The listing builds one solid part. Answer for the finished solid, in the listing's coordinates (mm). Coordinates: 2 decimals unless noted, no trailing zeros. Write each loop counter-clockwise with the first axis right and the second up, starting at its lowest first coordinate (ties: lowest second). Pieces come first, ordered by that corner, then holes. Notation, with made-up numbers: M 23.25,14.25 L 40.25,14.25 A36 cw 40.25,48.25 Z; hole C -40,77.5 d9. An arc over 180 degrees is marked long. Answer as CSV lines item,"result". Start each with the question number.
```python
from build123d import *

# Parameters (mm, degrees)
SKETCH_1_W             = 32.7
SKETCH_1_H             = 29
SKETCH_1_R             = 1.5
EXTRUDE_1_DEPTH        = 3
CHAMFER_1_SIZE         = 3
EXTRUDE_2_DEPTH        = 3
CHAMFER_2_SIZE         = 9.5
EXTRUDE_3_DEPTH        = 3
SKETCH_6_R             = 1.6
CUT_EXTRUDE_2_DEPTH    = 4
CUT_EXTRUDE_4_DEPTH    = 10
FILLET_2_R             = 1
FILLET_2_OF_MIRROR_1_R = 1


with BuildPart() as part:
    # 草图1 → 凸台-拉伸1 (new body)
    with BuildSketch(Plane.XY):
        Rectangle(SKETCH_1_W, SKETCH_1_H)
        with Locations((-14.35, -10)):
            Circle(SKETCH_1_R, mode=Mode.SUBTRACT)
        with Locations((-14.35, 10)):
            Circle(SKETCH_1_R, mode=Mode.SUBTRACT)
        with Locations((14.35, 10)):
            Circle(SKETCH_1_R, mode=Mode.SUBTRACT)
        with Locations((14.35, -10)):
            Circle(SKETCH_1_R, mode=Mode.SUBTRACT)
        with Locations((-14.35, 0)):
            Circle(SKETCH_1_R, mode=Mode.SUBTRACT)
        with Locations((14.35, 0)):
            Circle(SKETCH_1_R, mode=Mode.SUBTRACT)
    extrude(amount=EXTRUDE_1_DEPTH)

    # 倒角1
    chamfer_1_edges = [part.edges().sort_by_distance(p)[0] for p in [
        (16.35, -14.5, 1.5),
        (-16.35, -14.5, 1.5),
        (-16.35, 14.5, 1.5),
        (16.35, 14.5, 1.5),
    ]]
    chamfer(chamfer_1_edges, length=CHAMFER_1_SIZE)

    # 草图3 → 凸台-拉伸2 (add)
    with BuildSketch(Plane.XY.offset(3)):
        Polygon((-13.35, 14.5), (-68.5, 14.5), (-68.5, -14.5), (-13.35, -14.5), (-16.35, -11.5), (-16.35, 11.5), align=None)
        Polygon((68.5, 14.5), (13.35, 14.5), (16.35, 11.5), (16.35, -11.5), (13.35, -14.5), (68.5, -14.5), align=None)
    extrude(amount=-EXTRUDE_2_DEPTH)

    # 倒角2
    chamfer_2_edges = [part.edges().sort_by_distance(p)[0] for p in [
        (-68.5, -14.5, 1.5),
        (-68.5, 14.5, 1.5),
        (68.5, -14.5, 1.5),
        (68.5, 14.5, 1.5),
    ]]
    chamfer(chamfer_2_edges, length=CHAMFER_2_SIZE)

    # 草图4 → 凸台-拉伸3 (add)
    with BuildSketch(Plane(origin=(0, 0, 0), x_dir=(-1, 0, 0), z_dir=(0, 0, -1))):
        Polygon((-59, -14.5), (-53, -20.5), (53, -20.5), (59, -14.5), align=None)
    extrude(amount=-EXTRUDE_3_DEPTH)

    # 草图6 → 切除-拉伸2 (cut, through all)
    with BuildSketch(Plane(origin=(0, 0, 0), x_dir=(-1, 0, 0), z_dir=(0, 0, -1))):
        with Locations((-63.5, 0)):
            Circle(SKETCH_6_R)
    cut_extrude_2 = extrude(amount=-CUT_EXTRUDE_2_DEPTH, mode=Mode.SUBTRACT)

    # 草图7 → 切除-拉伸4 (cut)
    with BuildSketch(Plane(origin=(0, 0, 0), x_dir=(-1, 0, 0), z_dir=(0, 0, -1))):
        Polygon((-57, 11.5), (-65.5, 3), (-57.621320344, 3), (-49.121320344, 11.5), align=None)
        Polygon((-57.621320344, -3), (-65.5, -3), (-51, -17.5), (-43.121320344, -17.5), align=None)
        Polygon((-47.621320344, -3), (-53.378679656, -3), (-38.878679656, -17.5), (-33.121320344, -17.5), align=None)
        Polygon((-44.878679656, 11.5), (-53.378679656, 3), (-47.621320344, 3), (-39.121320344, 11.5), align=None)
        Polygon((-34.878679656, 11.5), (-43.378679656, 3), (-37.621320344, 3), (-29.121320344, 11.5), align=None)
        Polygon((-23.121320344, -17.5), (-37.621320344, -3), (-43.378679656, -3), (-28.878679656, -17.5), align=None)
        Polygon((-20, -8.5), (-25.5, -3), (-33.378679656, -3), (-20, -16.378679656), align=None)
        Polygon((-33.378679656, 3), (-25.5, 3), (-20, 8.5), (-20, 11.5), (-23, 11.5), (-24.878679656, 11.5), align=None)
    cut_extrude_4 = extrude(amount=-CUT_EXTRUDE_4_DEPTH, mode=Mode.SUBTRACT)

    # 圆角2
    fillet_2_edges = [part.edges().sort_by_distance(p)[0] for p in [
        (53.378679656, -3, 1.5),
        (47.621320344, -3, 1.5),
        (33.121320344, -17.5, 1.5),
        (38.878679656, -17.5, 1.5),
        (57.621320344, -3, 1.5),
        (43.121320344, -17.5, 1.5),
        (51, -17.5, 1.5),
        (65.5, -3, 1.5),
        (37.621320344, 3, 1.5),
        (43.378679656, 3, 1.5),
        (34.878679656, 11.5, 1.5),
        (29.121320344, 11.5, 1.5),
        (47.621320344, 3, 1.5),
        (53.378679656, 3, 1.5),
        (44.878679656, 11.5, 1.5),
        (39.121320344, 11.5, 1.5),
        (33.378679656, -3, 1.5),
        (25.5, -3, 1.5),
        (20, -8.5, 1.5),
        (20, -16.378679656, 1.5),
        (43.378679656, -3, 1.5),
        (37.621320344, -3, 1.5),
        (23.121320344, -17.5, 1.5),
        (28.878679656, -17.5, 1.5),
        (33.378679656, 3, 1.5),
        (24.878679656, 11.5, 1.5),
        (20, 11.5, 1.5),
        (20, 8.5, 1.5),
        (25.5, 3, 1.5),
        (57.621320344, 3, 1.5),
        (65.5, 3, 1.5),
        (57, 11.5, 1.5),
        (49.121320344, 11.5, 1.5),
    ]]
    fillet(fillet_2_edges, radius=FILLET_2_R)

    # 镜向1: 切除-拉伸2, 切除-拉伸4 across plane
    add(cut_extrude_2.mirror(Plane(origin=(0, 0, 0), x_dir=(0, 0, 1), z_dir=(1, 0, 0))), mode=Mode.SUBTRACT)
    add(cut_extrude_4.mirror(Plane(origin=(0, 0, 0), x_dir=(0, 0, 1), z_dir=(1, 0, 0))), mode=Mode.SUBTRACT)

    # 圆角2 of 镜向1
    fillet_2_of_mirror_1_edges = [part.edges().sort_by_distance(p)[0] for p in [
        (-53.378679656, -3, 1.5),
        (-47.621320344, -3, 1.5),
        (-33.121320344, -17.5, 1.5),
        (-38.878679656, -17.5, 1.5),
        (-57.621320344, -3, 1.5),
        (-43.121320344, -17.5, 1.5),
        (-51, -17.5, 1.5),
        (-65.5, -3, 1.5),
        (-37.621320344, 3, 1.5),
        (-43.378679656, 3, 1.5),
        (-34.878679656, 11.5, 1.5),
        (-29.121320344, 11.5, 1.5),
        (-47.621320344, 3, 1.5),
        (-53.378679656, 3, 1.5),
        (-44.878679656, 11.5, 1.5),
        (-39.121320344, 11.5, 1.5),
        (-33.378679656, -3, 1.5),
        (-25.5, -3, 1.5),
        (-20, -8.5, 1.5),
        (-20, -16.378679656, 1.5),
        (-43.378679656, -3, 1.5),
        (-37.621320344, -3, 1.5),
        (-23.121320344, -17.5, 1.5),
        (-28.878679656, -17.5, 1.5),
        (-33.378679656, 3, 1.5),
        (-24.878679656, 11.5, 1.5),
        (-20, 11.5, 1.5),
        (-20, 8.5, 1.5),
        (-25.5, 3, 1.5),
        (-57.621320344, 3, 1.5),
        (-65.5, 3, 1.5),
        (-57, 11.5, 1.5),
        (-49.121320344, 11.5, 1.5),
    ]]
    fillet(fillet_2_of_mirror_1_edges, radius=FILLET_2_OF_MIRROR_1_R)


solid = part.part
```
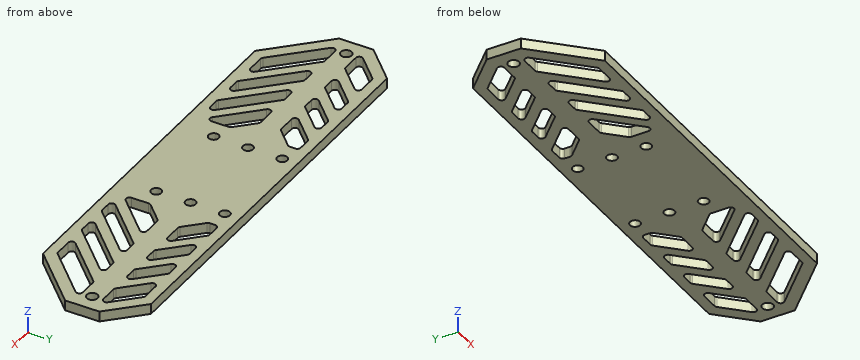
1) Each of these flat-tipped pins is pushed along its axis until it touches: P1, Ø1.8, axis at x = 14.35, y = 10, coming from the +Z side; P2, Ø1.5, axis at x = -54.5, z = 1, coming from the -Y side; P3, Ø0.5, axis at y = 9.5, z = 2, coming from the +X side. Where does it stop, or does it pass through?
2) Find the intervals of material crossed by line 1 (Y direction, x = 14.35, z = 0.85); line 2 (Y direction, x = -52, z = 1.2); line 3 (Y direction, x = 63.5, z = 2.1), in increasing order. Write a range as from..to.
3) The part is cut by section C-C (z = 1.05). Count the separate pieces of the cut face and the enclosed holes in it, then the cut area to 3 significant figures.
4) The part is cut by section A-A (y = 0). Determine the outline of the cut face in (x, z).
5) The part is cut by section B-B (x = 14.35). Determine the outline of the cut face in (y, z), then the cut area to 3 significant figures.
Completed:
1,P1,"through"
1,P2,"y = -19.75"
1,P3,"x = 64.25"
2,line 1,"-20.5..-11.5, -8.5..-1.5, 1.5..8.5, 11.5..14.5"
2,line 2,"-20.5..-16.5, -8.62..8.62, 11.5..14.5"
2,line 3,"-10..-5, -3.09..-1.6, 1.6..3.09, 5..10"
3,separate pieces,"1"
3,enclosed holes,"24"
3,area,"3,280 mm²"
4,outline,"M -68.5,0 L -65.1,0 L -65.1,3 L -68.5,3 Z; M -61.9,0 L -15.85,0 L -15.85,3 L -61.9,3 Z; M -12.85,0 L 12.85,0 L 12.85,3 L -12.85,3 Z; M 15.85,0 L 61.9,0 L 61.9,3 L 15.85,3 Z; M 65.1,0 L 68.5,0 L 68.5,3 L 65.1,3 Z"
5,outline,"M -20.5,0 L -11.5,0 L -11.5,3 L -20.5,3 Z; M -8.5,0 L -1.5,0 L -1.5,3 L -8.5,3 Z; M 1.5,0 L 8.5,0 L 8.5,3 L 1.5,3 Z; M 11.5,0 L 14.5,0 L 14.5,3 L 11.5,3 Z"
5,area,"78.0 mm²"
